Work out the finished part from the listing and answer in its coordinate system (mm). Face numbers are marked on the shaded views. A direction names the side the tool comes from. Coordinates: 2 decimals unless noted, no trailing zeros. Loops run counter-clockwise (first coordinate to the right, second up) from the corner with the lowest first, then second, coordinate; pieces in that order, holes last.
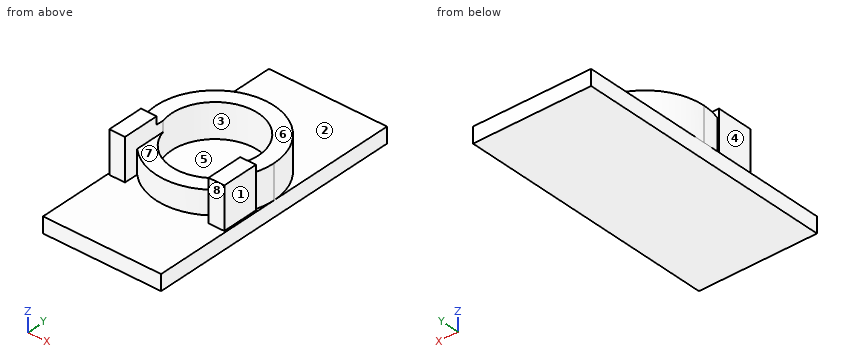
```python
from build123d import *

# Parameters (mm, degrees)
F0_R     = 8.3
F1_DEPTH = 6.5
F2_DEPTH = 8
F4_DEPTH = 2
F5_DEPTH = 3


with BuildPart() as f1:
    # F0 (on Top) → F1 (new body)
    with BuildSketch(Plane.XY):
        with BuildLine():
            ThreePointArc((10.6887791632, -3.666060556), (11.1461474184, -1.8583319746), (11.3, 0))
            ThreePointArc((11.3, 0), (6.7e-09, 11.3), (-11.3, 1.34e-08))
            ThreePointArc((-11.3, 1.34e-08), (-11.1461474195, -1.858331968), (-10.6887791632, -3.666060556))
            Line((-10.6887791632, -3.666060556), (-8, -3.666060556))
            Line((-8, -3.666060556), (-8, -7.9806014811))
            ThreePointArc((-8, -7.9806014811), (0, -11.3), (8, -7.9806014811))
            Line((8, -7.9806014811), (8, -3.666060556))
            Line((8, -3.666060556), (10.6887791632, -3.666060556))
        make_face()
        Circle(F0_R, mode=Mode.SUBTRACT)
    extrude(amount=F1_DEPTH)

    # F0 (on Top) → F2 (join)
    with BuildSketch(Plane.XY):
        with BuildLine():
            ThreePointArc((8, -7.9806014811), (9.5901737472, -5.9765012757), (10.6887791632, -3.666060556))
            Line((10.6887791632, -3.666060556), (8, -3.666060556))
            Line((8, -3.666060556), (8, -7.9806014811))
        make_face()
        with BuildLine():
            Line((11, -3.666060556), (10.6887791632, -3.666060556))
            ThreePointArc((10.6887791632, -3.666060556), (9.5901737472, -5.9765012757), (8, -7.9806014811))
            Line((8, -7.9806014811), (8, -10.666060556))
            Line((8, -10.666060556), (11, -10.666060556))
            Line((11, -10.666060556), (11, -3.666060556))
        make_face()
        with BuildLine():
            ThreePointArc((-8, -7.9806014811), (-9.5901737472, -5.9765012757), (-10.6887791632, -3.666060556))
            Line((-10.6887791632, -3.666060556), (-11, -3.666060556))
            Line((-11, -3.666060556), (-11, -10.666060556))
            Line((-11, -10.666060556), (-8, -10.666060556))
            Line((-8, -10.666060556), (-8, -7.9806014811))
        make_face()
        with BuildLine():
            Line((-8, -3.666060556), (-10.6887791632, -3.666060556))
            ThreePointArc((-10.6887791632, -3.666060556), (-9.5901737472, -5.9765012757), (-8, -7.9806014811))
            Line((-8, -7.9806014811), (-8, -3.666060556))
        make_face()
    extrude(amount=F2_DEPTH)

    # F3 (on face) → F4 (cut)
    with BuildSketch(Plane.XY.offset(6.5)):
        with BuildLine():
            Line((7.4464756765, -3.666060556), (-7.4464756765, -3.666060556))
            ThreePointArc((-7.4464756765, -3.666060556), (0, -8.3), (7.4464756765, -3.666060556))
        make_face()
        with BuildLine():
            Line((-7.4464756765, -3.666060556), (-8, -3.666060556))
            Line((-8, -3.666060556), (-8, -7.9806014811))
            ThreePointArc((-8, -7.9806014811), (-6.0175392622, -9.5644770494), (-3.7316420268, -10.666060556))
            Line((-3.7316420268, -10.666060556), (3.7316420268, -10.666060556))
            ThreePointArc((3.7316420268, -10.666060556), (6.0175392622, -9.5644770494), (8, -7.9806014811))
            Line((8, -7.9806014811), (8, -3.666060556))
            Line((8, -3.666060556), (7.4464756765, -3.666060556))
            ThreePointArc((7.4464756765, -3.666060556), (0, -8.3), (-7.4464756765, -3.666060556))
        make_face()
        with BuildLine():
            ThreePointArc((8, -7.9806014811), (6.0175392622, -9.5644770494), (3.7316420268, -10.666060556))
            Line((3.7316420268, -10.666060556), (8, -10.666060556))
            Line((8, -10.666060556), (8, -7.9806014811))
        make_face()
        with BuildLine():
            ThreePointArc((-3.7316420268, -10.666060556), (-6.0175392622, -9.5644770494), (-8, -7.9806014811))
            Line((-8, -7.9806014811), (-8, -10.666060556))
            Line((-8, -10.666060556), (-3.7316420268, -10.666060556))
        make_face()
        with BuildLine():
            Line((8, -10.666060556), (3.7316420268, -10.666060556))
            ThreePointArc((3.7316420268, -10.666060556), (1.8925532645, -11.1403878811), (0, -11.3))
            Line((0, -11.3), (8, -11.3))
            Line((8, -11.3), (8, -10.666060556))
        make_face()
        with BuildLine():
            Line((3.7316420268, -10.666060556), (-3.7316420268, -10.666060556))
            ThreePointArc((-3.7316420268, -10.666060556), (-1.8925532645, -11.1403878811), (0, -11.3))
            ThreePointArc((0, -11.3), (1.8925532645, -11.1403878811), (3.7316420268, -10.666060556))
        make_face()
        with BuildLine():
            Line((-3.7316420268, -10.666060556), (-8, -10.666060556))
            Line((-8, -10.666060556), (-8, -11.3))
            Line((-8, -11.3), (0, -11.3))
            ThreePointArc((0, -11.3), (-1.8925532645, -11.1403878811), (-3.7316420268, -10.666060556))
        make_face()
        with BuildLine():
            ThreePointArc((8, -2.2113344387), (7.7574132109, -2.951701251), (7.4464756765, -3.666060556))
            Line((7.4464756765, -3.666060556), (8, -3.666060556))
            Line((8, -3.666060556), (8, -2.2113344387))
        make_face()
        with BuildLine():
            Line((-8, -2.2113344387), (-8, -3.666060556))
            Line((-8, -3.666060556), (-7.4464756765, -3.666060556))
            ThreePointArc((-7.4464756765, -3.666060556), (-7.7574132109, -2.951701251), (-8, -2.2113344387))
        make_face()
        with BuildLine():
            ThreePointArc((-8, -2.2113344387), (-7.7574132109, -2.951701251), (-7.4464756765, -3.666060556))
            Line((-7.4464756765, -3.666060556), (7.4464756765, -3.666060556))
            ThreePointArc((7.4464756765, -3.666060556), (7.7574132109, -2.951701251), (8, -2.2113344387))
            Line((8, -2.2113344387), (-8, -2.2113344387))
        make_face()
    extrude(amount=-F4_DEPTH, mode=Mode.SUBTRACT)

    # F0 (on Top) → F5 (join)
    with BuildSketch(Plane.XY):
        with BuildLine():
            ThreePointArc((10.6887791632, -3.666060556), (11.1461474184, -1.8583319746), (11.3, 0))
            ThreePointArc((11.3, 0), (6.7e-09, 11.3), (-11.3, 1.34e-08))
            ThreePointArc((-11.3, 1.34e-08), (-11.1461474195, -1.858331968), (-10.6887791632, -3.666060556))
            Line((-10.6887791632, -3.666060556), (-8, -3.666060556))
            Line((-8, -3.666060556), (-8, -7.9806014811))
            ThreePointArc((-8, -7.9806014811), (0, -11.3), (8, -7.9806014811))
            Line((8, -7.9806014811), (8, -3.666060556))
            Line((8, -3.666060556), (10.6887791632, -3.666060556))
        make_face()
        Circle(F0_R, mode=Mode.SUBTRACT)
        with BuildLine():
            ThreePointArc((8, -7.9806014811), (9.5901737472, -5.9765012757), (10.6887791632, -3.666060556))
            Line((10.6887791632, -3.666060556), (8, -3.666060556))
            Line((8, -3.666060556), (8, -7.9806014811))
        make_face()
        with BuildLine():
            Line((11, -3.666060556), (10.6887791632, -3.666060556))
            ThreePointArc((10.6887791632, -3.666060556), (9.5901737472, -5.9765012757), (8, -7.9806014811))
            Line((8, -7.9806014811), (8, -10.666060556))
            Line((8, -10.666060556), (11, -10.666060556))
            Line((11, -10.666060556), (11, -3.666060556))
        make_face()
        with BuildLine():
            Line((-8, -3.666060556), (-10.6887791632, -3.666060556))
            ThreePointArc((-10.6887791632, -3.666060556), (-9.5901737472, -5.9765012757), (-8, -7.9806014811))
            Line((-8, -7.9806014811), (-8, -3.666060556))
        make_face()
        with BuildLine():
            ThreePointArc((-8, -7.9806014811), (-9.5901737472, -5.9765012757), (-10.6887791632, -3.666060556))
            Line((-10.6887791632, -3.666060556), (-11, -3.666060556))
            Line((-11, -3.666060556), (-11, -10.666060556))
            Line((-11, -10.666060556), (-8, -10.666060556))
            Line((-8, -10.666060556), (-8, -7.9806014811))
        make_face()
        with BuildLine():
            Line((11.3, -25), (11.3, 0))
            ThreePointArc((11.3, 0), (11.1461474184, -1.8583319746), (10.6887791632, -3.666060556))
            Line((10.6887791632, -3.666060556), (11, -3.666060556))
            Line((11, -3.666060556), (11, -10.666060556))
            Line((11, -10.666060556), (8, -10.666060556))
            Line((8, -10.666060556), (8, -7.9806014811))
            ThreePointArc((8, -7.9806014811), (0, -11.3), (-8, -7.9806014811))
            Line((-8, -7.9806014811), (-8, -10.666060556))
            Line((-8, -10.666060556), (-11, -10.666060556))
            Line((-11, -10.666060556), (-11, -3.666060556))
            Line((-11, -3.666060556), (-10.6887791632, -3.666060556))
            ThreePointArc((-10.6887791632, -3.666060556), (-11.1461474195, -1.858331968), (-11.3, 1.34e-08))
            Line((-11.3, 1.34e-08), (-11.3, -25))
            Line((-11.3, -25), (11.3, -25))
        make_face()
        with BuildLine():
            ThreePointArc((-11.3, 1.34e-08), (6.7e-09, 11.3), (11.3, 0))
            Line((11.3, 0), (11.3, 25))
            Line((11.3, 25), (-11.3, 25))
            Line((-11.3, 25), (-11.3, 1.34e-08))
        make_face()
        Circle(F0_R)
    extrude(amount=-F5_DEPTH)


solid = f1.part
```
1. A cutting plane is placed at A-A, the plane z = 5. Give the vertices of the cut face in (x, y), then the cut area to 3 significant figures.
2. For the marked faces 4, 5, 6, 7 and 8, determine the directions among +Z, -Z, +X, -X, +Y, -Y from which every point of the face is accessible in a straight line to the end or side of a thin tool.
3. A cutting plane is placed at C-C, the plane y = 15.5. Give the vertices of the cut face in (x, z), then the cut area to 3 significant figures.
4. Each of these flat-tipped pins is pushed along its axis until it touches: P1, Ø3, axis at x = -9, z = 2.5, coming from the +Y side; P2, Ø2.5, axis at x = -10, z = 2.5, coming from the -Y side; P3, Ø5, axis at x = -0.5, y = -1, coming from the +Z side. Where does it stop, or does it pass through?
5. A cutting plane is placed at B-B, the plane x = 0. Give the vertices of the cut face in (y, z), then the cut area to 3 significant figures.
6. Determine the mould class of the marked faces 1, 2 and 3 for opening direction X: released by +X, released by -X, zero draft, split by the parting line, or undercut.
7. Straight lines are drawn through the part: probe 1 along Y at (x, z) = (0, 1.75); probe 2 along Z at (x, y) = (-3.5, -15); probe 3 along X at (y, z) = (-4, 6.75). For each, find the intervals that lie inside material, in ascending order.
Answers below:
1. outline: (-11, -10.67) - (-8, -10.67) - (-8, -2.21) arc R8.3 cw (long way) to (8, -2.21) - (8, -10.67) - (11, -10.67) - (11, -3.67) - (10.69, -3.67) arc R11.3 ccw (long way) to (-10.69, -3.67) - (-11, -3.67) - close
1. area: 156 mm2
2. face 4: +Z, -X, -Y
2. face 5: +Z
2. face 6: +Z, +X, -X, +Y
2. face 7: +Z, -Y
2. face 8: +Z, +X, -Y
3. outline: (-11.3, -3) - (11.3, -3) - (11.3, 0) - (-11.3, 0) - close
3. area: 67.8 mm2
4. P1: stops at y = 8.45
4. P2: stops at y = -10.67
4. P3: stops at z = 0
5. outline: (-25, -3) - (25, -3) - (25, 0) - (11.3, 0) - (11.3, 6.5) - (8.3, 6.5) - (8.3, 0) - (-8.3, 0) - (-8.3, 4.5) - (-11.3, 4.5) - (-11.3, 0) - (-25, 0) - close
5. area: 183 mm2
6. face 1: released by +X
6. face 2: zero draft
6. face 3: undercut
7. probe 1: y = -11.3 to -8.3, 8.3 to 11.3
7. probe 2: z = -3 to 0
7. probe 3: x = -11 to -8, 8 to 11
